Autodesk Inventor part; units mm, degrees
ref_plane "YZ Plane" through (0, 0, 0) normal (1, 0, 0) x (0, 1, 0)
ref_plane "XZ Plane" through (0, 0, 0) normal (0, 1, 0) x (-1, 0, 0)
ref_plane "XY Plane" through (0, 0, 0) normal (0, 0, 1) x (1, 0, 0)
sketch "草图1" plane through (0, 0, 0) normal (0, 0, 1) x (1, 0, 0)
  arc A0 (-6.7099, -1.9944) -> (-6.7099, 1.9944) centre (0, 0) ccw
  line L0 (-6.7099, -1.9944) -> (-10.6762, -1.9944)
  line L1 (-10.6762, -1.9944) -> (-10.6762, 1.9944)
  line L2 (-10.6762, 1.9944) -> (-6.7099, 1.9944)
  line L3 (-2.516, -5.9831) -> (-10.6762, 1.9944) construction
  line L4 (-10.6762, -1.9944) -> (-0.0773, -1.9944) construction
  circle A1 centre (0, 0) radius 1.6
  point P0 (-6.5961, -1.9944)
  dimension "d0" = 7
  dimension "d1" = 3.2
extrude "拉伸1" add sketch "草图1" along normal blind 5
sketch "草图2" plane through (0, 0, 0) normal (0, 0, -1) x (-1, 0, 0)
  circle A0 centre (0, 0) radius 5.25
  dimension "d4" = 10.5
extrude "拉伸2" cut sketch "草图2" against normal blind 1.5
sketch "草图3" plane through (0, 0, 5) normal (0, 0, 1) x (1, 0, 0)
  circle A0 centre (0, 0) radius 3.25
  dimension "d7" = 6.5
extrude "拉伸3" cut sketch "草图3" against normal blind 1.5
fillet "圆角1" radius 1 1 edges at (-3.25, 0, 3.5)
properties part number "编码器模型"
Input: part model. Units: mm. Frame: model coordinates. A direction names the side the tool comes from. Give positions to 0.01 mm unless a question says otherwise; leave off trailing zeros. Order: outer loops, then holes, each group sorted by start corner. A loop starts at its lowest first (then second) coordinate and runs counter-clockwise, first axis right, second up. Notation, with made-up numbers: M 28.5,74 L 72.5,74 A30 cw 72.5,113 Z; hole C 86,76.25 d5. An arc over 180 degrees is marked long. Return JSON: item names as keys, results as strings.
Item 1: Cut plane C-C (y = 0). Return loops of the section in (x, z).
Solutions:
{"outline": "M -10.68,0 L -5.25,0 L -5.25,1.5 L -1.6,1.5 L -1.6,3.5 L -2.25,3.5 A1 cw -3.25,4.5 L -3.25,5 L -10.68,5 Z; M 1.6,1.5 L 5.25,1.5 L 5.25,0 L 7,0 L 7,5 L 3.25,5 L 3.25,4.5 A1 cw 2.25,3.5 L 1.6,3.5 Z"}
Item 2: First-contact query: P1, Ø1.2, axis at x = -8, z = 3.5, coming from the +Y side; P2, Ø1.3, axis at x = -0.5, y = 1, coming from the +Z side; P3, Ø3, axis at x = -0.5, y = 2.5, coming from the -Z side. Flat tips, straight axial feed; report the tip coordinate or a pass-through.
Solutions:
{"P1": "y = 1.99", "P2": "z = 3.5", "P3": "z = 1.5"}
Item 3: Cut plane D-D (y = -5). Return loops of the section in (x, z), then the cut area to 3 significant figures.
Solutions:
{"outline": "M -4.9,0 L -1.6,0 L -1.6,1.5 L 1.6,1.5 L 1.6,0 L 4.9,0 L 4.9,5 L -4.9,5 Z", "area": "44.2 mm^2"}
Item 4: Cut plane B-B (z = 2.85). Return loops of the section in (x, y), then the cut area to 3 significant figures.
Solutions:
{"outline": "M -10.68,-1.99 L -6.71,-1.99 A7 ccw long -6.71,1.99 L -10.68,1.99 Z; hole C 0,0 d3.2", "area": "161 mm^2"}
Item 5: Pull-direction query (X, two-part tool) for faces 1 (the flat face through (-4, 0, 5)), 2 (the cylindrical face through (7, 0, 2)), 3 (the flat face through (-2, 0, 3.5)); classes: +X half, -X half, draft (parallel to the pull), parting line (faces both ways), or undercut.
Solutions:
{"face 1": "draft", "face 2": "parting line", "face 3": "undercut"}
Item 6: Access query for faces 4 (the cylindrical face through (-5, 1.6, 0.7)), 5 (the flat face through (-9, 1.994, 2)), 6 (the flat face through (-9, -1.994, 2)). Directions: +Z, -Z, +X, -X, +Y, -Y. A direction counts if a zero-diameter tool reaches every point of the face in a straight line with its end or side. Return the directions, or none.
Solutions:
{"face 4": "-Z", "face 5": "+Z, -Z, -X, +Y", "face 6": "+Z, -Z, -X, -Y"}
Item 7: Ray query, probe 1 along Y at (x, z) = (0, 4.75); probe 2 along Y at (x, z) = (0, 2.4); probe 3 along Z at (x, y) = (2.75, 2.25). Return the intervals inside material, ascending.
Solutions:
{"probe 1": "-7 to -3.25, 3.25 to 7", "probe 2": "-7 to -1.6, 1.6 to 7", "probe 3": "1.5 to 5"}
Item 8: Cut plane A-A (x = 0). Return loops of the section in (y, z), then the cut area to 3 significant figures.
Solutions:
{"outline": "M -7,0 L -5.25,0 L -5.25,1.5 L -1.6,1.5 L -1.6,3.5 L -2.25,3.5 A1 cw -3.25,4.5 L -3.25,5 L -7,5 Z; M 1.6,1.5 L 5.25,1.5 L 5.25,0 L 7,0 L 7,5 L 3.25,5 L 3.25,4.5 A1 cw 2.25,3.5 L 1.6,3.5 Z", "area": "38.5 mm^2"}
